```python
from build123d import *

# Parameters (mm, degrees)
SKETCH1_W             = 96
SKETCH1_H             = 56
BOSS_EXTRUDE1_DEPTH   = 3.8
SKETCH2_W             = 96
SKETCH2_H             = 35
BOSS_EXTRUDE2_DEPTH   = 2.3
CUT_EXTRUDE1_DEPTH    = 3.3
SKETCH4_R             = 1.5
CUT_EXTRUDE2_DEPTH    = 3.3
SKETCH5_W             = 96
SKETCH5_H             = 2
BOSS_EXTRUDE3_DEPTH   = 11.5
BOSS_EXTRUDE5_DEPTH   = 48
LPATTERN1_COUNT       = 6
LPATTERN1_PITCH       = 7.7
SKETCH8_W             = 28
SKETCH8_H             = 2.3
CUT_EXTRUDE3_DEPTH    = 0.7
M3X0_5_TAPPED_HOLE1_D = 2.5
LPATTERN2_COUNT       = 2
LPATTERN2_PITCH       = 38.5


with BuildPart() as part:
    # Sketch1 → Boss-Extrude1 (new body)
    with BuildSketch(Plane(origin=(0, 0, 0), x_dir=(1, 0, 0), z_dir=(0, 1, 0))):
        Rectangle(SKETCH1_W, SKETCH1_H)
    extrude(amount=BOSS_EXTRUDE1_DEPTH)

    # Sketch2 → Boss-Extrude2 (add)
    with BuildSketch(Plane(origin=(0, 0, -28), x_dir=(-1, 0, 0), z_dir=(0, 0, -1))):
        with Locations((0, 6)):
            Rectangle(SKETCH2_W, SKETCH2_H)
    extrude(amount=-BOSS_EXTRUDE2_DEPTH)

    # Sketch3 → Cut-Extrude1 (cut, through all)
    with BuildSketch(Plane(origin=(0, 0, -25.7), x_dir=(-1, 0, 0), z_dir=(0, 0, -1))):
        with BuildLine():
            Line((-52.45, 14), (-43.55, 14))
            ThreePointArc((-43.55, 14), (-41.3, 11.75), (-43.55, 9.5))
            Line((-43.55, 9.5), (-52.45, 9.5))
            ThreePointArc((-52.45, 9.5), (-54.7, 11.75), (-52.45, 14))
        make_face()
    cut_extrude1 = extrude(amount=CUT_EXTRUDE1_DEPTH, mode=Mode.SUBTRACT)

    # Sketch4 → Cut-Extrude2 (cut, through all)
    with BuildSketch(Plane.XY.offset(-25.7)):
        with Locations((39.5, 17.7)):
            Circle(SKETCH4_R)
    cut_extrude2 = extrude(amount=-CUT_EXTRUDE2_DEPTH, mode=Mode.SUBTRACT)

    # Mirror1: Cut-Extrude1, Cut-Extrude2 across plane
    add(cut_extrude1.mirror(Plane(origin=(0, 0, 0), x_dir=(0, 0, 1), z_dir=(1, 0, 0))), mode=Mode.SUBTRACT)
    add(cut_extrude2.mirror(Plane(origin=(0, 0, 0), x_dir=(0, 0, 1), z_dir=(1, 0, 0))), mode=Mode.SUBTRACT)

    # Sketch5 → Boss-Extrude3 (add)
    with BuildSketch(Plane(origin=(0, 0, 0), x_dir=(1, 0, 0), z_dir=(0, 1, 0))):
        with Locations((0, -27)):
            Rectangle(SKETCH5_W, SKETCH5_H)
    extrude(amount=-BOSS_EXTRUDE3_DEPTH)

    # Sketch7 → Boss-Extrude5 (add, symmetric)
    with BuildSketch(Plane(origin=(0, 0, 0), x_dir=(0, 0, -1), z_dir=(1, 0, 0))):
        Polygon((-21.7, 0), (-21.2, -11.5), (-20.5, -11.5), (-20, 0), align=None)
    boss_extrude5 = extrude(amount=BOSS_EXTRUDE5_DEPTH, both=True)

    # LPattern1: Boss-Extrude5 ×6
    with Locations(*[(0, 0, -i * LPATTERN1_PITCH) for i in range(1, LPATTERN1_COUNT)]):
        add(boss_extrude5)

    # Sketch8 → Cut-Extrude3 (cut)
    with BuildSketch(Plane(origin=(0, 23.5, 0), x_dir=(1, 0, 0), z_dir=(0, 1, 0))):
        with Locations((0, 26.85)):
            Rectangle(SKETCH8_W, SKETCH8_H)
    extrude(amount=-CUT_EXTRUDE3_DEPTH, mode=Mode.SUBTRACT)

    # M3x0.5 Tapped Hole1 (through all)
    with Locations(Plane(origin=(0, 3.8, 0), x_dir=(1, 0, 0), z_dir=(0, 1, 0))):
        with Locations((-34.3, -17.3), (34.3, -17.3)):
            m3x0_5_tapped_hole1 = Hole(M3X0_5_TAPPED_HOLE1_D / 2)

    # LPattern2: M3x0.5 Tapped Hole1 ×2
    with Locations(*[(0, 0, -i * LPATTERN2_PITCH) for i in range(1, LPATTERN2_COUNT)]):
        add(m3x0_5_tapped_hole1, mode=Mode.SUBTRACT)


solid = part.part
```
Check sheet for the modelled part. Datum: model origin and axes. Units: mm. A direction names the side the tool comes from. Round coordinates to 2 decimals unless told otherwise and drop trailing zeros. Order: outer loops, then holes, each group sorted by start corner. A loop starts at its lowest first (then second) coordinate and runs counter-clockwise, first axis right, second up. Notation, with made-up numbers: (15, 7.25) - (28, 7.25) arc R8 ccw to (28, 14.25) - close; hole circle Ø7 at (-10, 46). An arc over 180 degrees is marked (long way). Write item = value, one per line.
Q1. Section check A-A (z = 17.3). Record the boundary of the cut face in (x, y).
Computed:
outline = (-48, 0) - (-35.55, 0) - (-35.55, 3.8) - (-48, 3.8) - close; (-33.05, 0) - (33.05, 0) - (33.05, 3.8) - (-33.05, 3.8) - close; (35.55, 0) - (48, 0) - (48, 3.8) - (35.55, 3.8) - close
Q2. Section check B-B (y = 17.7). Record the boundary of the cut face in (x, z).
Computed:
outline = (-48, -28) - (-41, -28) - (-41, -25.7) - (-48, -25.7) - close; (-38, -28) - (38, -28) - (38, -25.7) - (-38, -25.7) - close; (41, -28) - (48, -28) - (48, -25.7) - (41, -25.7) - close
Q3. Draft check along X on faces 1 (the face through (1, 14, -25.7)), 2 (the face through (38.39, 18.71, -26.83)), 3 (the face through (-38.39, 18.71, -26.83)), 4 (the face through (41.3, 11.8, -26.8)). Enter one of: pulls with the +X half, pulls with the -X half, needs draft (parallel to the pull), parting line crosses it, or undercut.
Computed:
face_1 = needs draft
face_2 = undercut
face_3 = undercut
face_4 = pulls with the +X half
Q4. Thickness scan on line 1 along Z through (x, y) = (34.3, 1.4); line 2 along X through (y, z) = (0.9, -21.2); line 3 along Y through (x, z) = (-39.5, -27). Record the ranges inside material, lowest first.
Computed:
line_1 = -28 to -22.45, -19.95 to 16.05, 18.55 to 28
line_2 = -48 to -35.55, -33.05 to 33.05, 35.55 to 48
line_3 = -11.5 to 16.2, 19.2 to 23.5
Q5. Go/stop test with flat-tipped pins: pin 1 (4 mm diameter, centred on x = -8.5, y = 7.5, fed in from +Z); pin 2 (3 mm diameter, centred on x = 5.5, z = 10.5, fed in from -Y); pin 3 (2 mm diameter, centred on x = 8.5, z = 6.5, fed in from +Y); pin 4 (2 mm diameter, centred on x = -34.3, z = -21.2, fed in from +Y). Record where each tip stops, or that it passes through.
Computed:
pin_1 = -25.7
pin_2 = 0
pin_3 = 3.8
pin_4 = through
Q6. Section check D-D (y = -7). State how many separate pieces and enclosed holes the cut face has, and give its area (3 significant figures).
Computed:
separate_pieces = 8
enclosed_holes = 0
area = 1,040 mm^2
Q7. Tool access check on faces 5 (the face through (1, 6, -28)), 6 (the face through (-46, 9.5, -27)), 7 (the face through (-1, -6, 26)). Record the directions out of +Z, -Z, +X, -X, +Y, -Y that give a thin tool (end or side, any length) a straight path to the whole face; none if there is none.
Computed:
face_5 = -Z, +X, -X, +Y, -Y
face_6 = +Z, -Z, -X
face_7 = +X, -X, -Y
